```python
from build123d import *

# Parameters (mm, degrees)
CORTAR_EXTRUIR1_DEPTH      = 70
CORTAR_EXTRUIR1_DEPTH_BACK = 70
CROQUIS2_W                 = 77.259476102
CROQUIS2_H                 = 391.167224263
CHAFL_N1_SIZE              = 10
REDONDEO1_R                = 10


with BuildPart() as part:
    # Croquis1 → Revolución1 (revolve)
    with BuildSketch(Plane.XY):
        with BuildLine():
            Line((-28, 35), (-16, 35))
            Line((-16, 35), (-16, 25))
            Line((-16, 25), (-25, 25))
            Line((-25, 25), (-25, 15))
            Line((-25, 15), (-16, 15))
            Line((-16, 15), (-16, -15))
            Line((-16, -15), (-25, -15))
            Line((-25, -15), (-25, -25))
            Line((-25, -25), (-16, -25))
            Line((-16, -25), (-16, -35))
            Line((-16, -35), (-29.067033725, -35))
            add(Edge.make_bspline(
                [(-47, -350), (-74.627383194, -246.893202238), (-41.199250834, -146.705952206), (-29.067033725, -35)],
                knots=[0, 0, 0, 0, 0.830416843, 0.830416843, 0.830416843, 0.830416843], degree=3))
            Line((-47, -350), (-50, -350))
            add(Edge.make_bspline(
                [(-28, 35), (-28, -105.90833009), (-83.269295344, -225.837299443), (-50, -350)],
                knots=[0, 0, 0, 0, 1, 1, 1, 1], degree=3))
        make_face()
    revolve(axis=Axis((0, 50, 0), (0, -1, 0)))

    # Croquis2 → Cortar-Extruir1 (cut, two sides: drawn at the far end of the back side and taken through both)
    with BuildSketch(Plane(origin=(0, 0, 0), x_dir=(0, 0, -1), z_dir=(1, 0, 0)).offset(-CORTAR_EXTRUIR1_DEPTH_BACK)):
        with Locations((-38.629738051, -154.416387869)):
            Rectangle(CROQUIS2_W, CROQUIS2_H)
    extrude(amount=CORTAR_EXTRUIR1_DEPTH + CORTAR_EXTRUIR1_DEPTH_BACK, mode=Mode.SUBTRACT)

    # Chaflán1
    # the kernel refuses this chamfer: 10 mm, written as the material it takes off along each edge
    with BuildSketch(Plane(origin=(0, 35, 0), x_dir=(-0.5990091787085334, 0, 0.8007421581401396), z_dir=(0.8007421581401396, 0, 0.5990091787085334))) as chafl_n1_piece_1:
        with BuildLine():
            Line((28 - CHAFL_N1_SIZE, 0), (28.093218581, 10.093218581))
            ThreePointArc((28.093218581, 10.093218581), (28.024813117, 5.189585851), (28, 0))
            Line((28, 0), (28 - CHAFL_N1_SIZE, 0))
        make_face()
    revolve(axis=Axis((0, 35, 0), (0, -1, 0)), revolution_arc=286.402063585, mode=Mode.SUBTRACT)

    # Redondeo1
    # the kernel refuses this fillet: 10 mm, written as the material it takes off along each edge
    with BuildSketch(Plane(origin=(0, 24.906781419, 0), x_dir=(-0.9366579963611824, 0, 0.35024533951596737), z_dir=(0.35024533951596737, 0, 0.9366579963611824))) as redondeo1_piece_1:
        with BuildLine():
            CenterArc((18.183388392, 4.232305435), REDONDEO1_R, 315, 43.547945444)
            Line((28.180177192, 3.978901233), (28.380112968, 3.973833149))
            ThreePointArc((28.380112968, 3.973833149), (28.333165909, 1.985155745), (28.293184954, -0.003667366))
            Line((28.293184954, -0.003667366), (28.234639937, -0.141421356))
            Line((28.234639937, -0.141421356), (25.39587756, -2.980183733))
            Line((25.39587756, -2.980183733), (25.254456204, -2.838762377))
        make_face()
    revolve(axis=Axis((0, 24.906781419, 0), (0, -1, 0)), revolution_arc=221.004643811, mode=Mode.SUBTRACT)
    with BuildSketch(Plane(origin=(0, 35, 0), x_dir=(-0.8695683162103452, 0, 0.4938126602701729), z_dir=(0.4938126602701729, 0, 0.8695683162103452))) as redondeo1_piece_2:
        with BuildLine():
            CenterArc((13.554140544, 9.696276168), REDONDEO1_R, 284.157365729, 30.842634271)
            Line((20.625208356, 2.625208356), (20.766629712, 2.483787))
            Line((20.766629712, 2.483787), (18.141421356, -0.141421356))
            Line((18.141421356, -0.141421356), (18, -0.2))
            ThreePointArc((18, -0.2), (17, -0.2), (16.048917189, -0.193925523))
            Line((16.048917189, -0.193925523), (16, 0))
        make_face()
    revolve(axis=Axis((0, 35, 0), (0, -1, 0)), revolution_arc=239.182972496, mode=Mode.SUBTRACT)


solid = part.part
```
Part model, mm, in its own coordinate system. A direction names the side the tool comes from. Round coordinates to 2 decimals unless told otherwise and drop trailing zeros.
Item 1: Which spindle directions (+Z, -Z, +X, -X, +Y, -Y) get a long thin tool onto all of the face, cutting with end or side? Do faces 4 (the cylindrical face through (-0.55, -20.07, -24.994)), 5 (the conical face through (0, 32, -21)). Say none if no direction does.
Results:
face 4: +Z
face 5: -Z, +Y
Item 2: Probe L1, parallel to Y at x = -24, z = -5.5; L2, parallel to X at y = -94.5, z = -17; L3, parallel to X at y = -268, z = -3.5. List the from-to ranges inside material, lowest first.
Results:
L1: y = -35 to -25, -15 to 15, 25 to 28.38
L2: x = -36.48 to -33.14, 33.14 to 36.48
L3: x = -60.54 to -57.53, 57.53 to 60.54
Item 3: Two-plate mould, pull along Y, no slides. Class faces 1 (the flat face through (0, -35, -18)), 2 (the flat face through (38.5, -101.4, 0)), 3 (the cylindrical face through (-0.55, 19.93, -24.994)): +Y half, -Y half, draft (parallel to the pull), parting line (faces both ways), or undercut.
Results:
face 1: -Y half
face 2: draft
face 3: undercut
Item 4: Drop flat-ended pins along their axis: pin 1 Ø4 at (x, y) = (19, -28) entering from -Z; pin 2 Ø23.5 at (x, z) = (5.5, -15) entering from -Y; pin 3 Ø1.5 at (x, z) = (-18.5, -20) entering from +Y. Give the stop position or say it passes through.
Results:
pin 1: stops at z = -26.35
pin 2: stops at y = -35
pin 3: stops at y = 26.24
